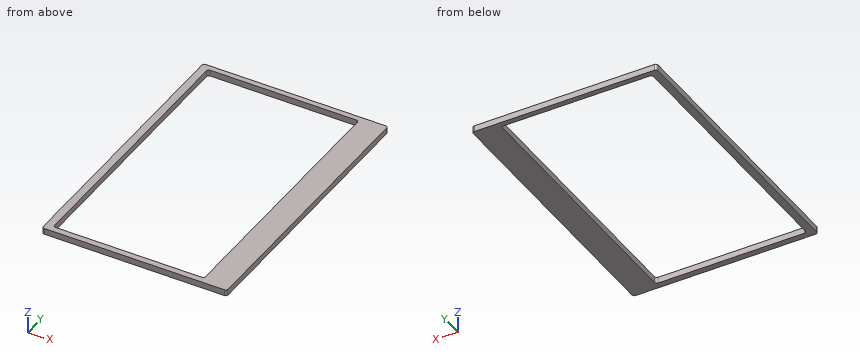
```python
from build123d import *

# Parameters (mm, degrees)
BOX001_W     = 98
BOX001_H     = 173.5
BOX001_DEPTH = 10
FILLET_R     = 1.5
BOX_W        = 120
BOX_H        = 181
BOX_DEPTH    = 4
FILLET001_R  = 1.5


with BuildPart() as fillet_body:
    # Box001 → Box001 (new body)
    with BuildSketch(Plane(origin=(7, 4, 0), x_dir=(1, 0, 0), z_dir=(0, 0, 1))):
        with Locations((49, 86.75)):
            Rectangle(BOX001_W, BOX001_H)
    extrude(amount=BOX001_DEPTH)

    # Fillet
    fillet_edges = [fillet_body.edges().sort_by_distance(p)[0] for p in [
        (7, 4, 5),
        (7, 177.5, 5),
        (105, 4, 5),
        (105, 177.5, 5),
    ]]
    fillet(fillet_edges, radius=FILLET_R)


with BuildPart() as cut:
    # Box → Box (new body)
    with BuildSketch(Plane(origin=(2, 0, 0), x_dir=(1, 0, 0), z_dir=(0, 0, 1))):
        with Locations((60, 90.5)):
            Rectangle(BOX_W, BOX_H)
    extrude(amount=BOX_DEPTH)

    # Fillet001
    fillet001_edges = [cut.edges().sort_by_distance(p)[0] for p in [
        (2, 0, 2),
        (2, 181, 2),
        (122, 0, 2),
        (122, 181, 2),
    ]]
    fillet(fillet001_edges, radius=FILLET001_R)

    # Cut: cut Fillet body
    add(fillet_body.part, mode=Mode.SUBTRACT)


solid = cut.part
```
Model file for the job. Use its own axes, mm. Round coordinates to 2 decimals unless told otherwise and drop trailing zeros. Order: outer loops, then holes, each group sorted by start corner. A loop starts at its lowest first (then second) coordinate and runs counter-clockwise, first axis right, second up. Notation, with made-up numbers: M 66.25,59.5 L 107.25,59.5 A19 ccw 107.25,80.5 Z; hole C 11,18 d9. An arc over 180 degrees is marked long. Use CSV: the item, a comma, the result in double quotes.
Item 1: Probe probe 1 along X at (y, z) = (51, 1.5); probe 2 along Y at (x, z) = (94, 2.4). List the from-to ranges inside material, lowest first.
Worked answers:
probe 1,"2 to 7, 105 to 122"
probe 2,"0 to 4, 177.5 to 181"
Item 2: Saw through at B-B (y = 65). List the corners of the cut face in (x, z).
Worked answers:
outline,"M 2,0 L 7,0 L 7,4 L 2,4 Z; M 105,0 L 122,0 L 122,4 L 105,4 Z"
Item 3: Saw through at C-C (x = 42.5). List the corners of the cut face in (y, z).
Worked answers:
outline,"M 0,0 L 4,0 L 4,4 L 0,4 Z; M 177.5,0 L 181,0 L 181,4 L 177.5,4 Z"
Item 4: Saw through at A-A (z = 3.05). List the corners of the cut face in (x, y), plus the area to 3 significant figures.
Worked answers:
outline,"M 2,1.5 A1.5 ccw 3.5,0 L 120.5,0 A1.5 ccw 122,1.5 L 122,179.5 A1.5 ccw 120.5,181 L 3.5,181 A1.5 ccw 2,179.5 Z; hole M 7,5.5 A1.5 ccw 8.5,4 L 103.5,4 A1.5 ccw 105,5.5 L 105,176 A1.5 ccw 103.5,177.5 L 8.5,177.5 A1.5 ccw 7,176 Z"
area,"4,720 mm²"
